The listing builds one solid part. Answer for the finished solid, in the listing's coordinates (mm). Face numbers are marked on the shaded views. A direction names the side the tool comes from. Coordinates: 2 decimals unless noted, no trailing zeros. Order: outer loops, then holes, each group sorted by start corner. A loop starts at its lowest first (then second) coordinate and runs counter-clockwise, first axis right, second up. Notation, with made-up numbers: (27, 21) -> (55, 21) arc R7 cw to (55, 30) -> close; hole circle Ø1 at (55, 55). An arc over 180 degrees is marked (long way). Return JSON: item names as keys, results as strings.
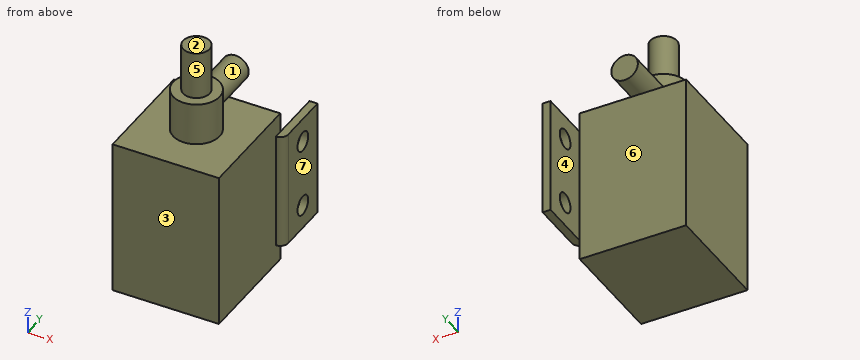
Autodesk Fusion 360 part; units mm, degrees
sketch "Sketch1" plane through (0, 0, 0) normal (0, 0, 1) x (1, 0, 0)
  line L0 (0, 0) -> (20, 0)
  line L1 (20, 0) -> (20, 21)
  line L2 (20, 21) -> (0, 21)
  line L3 (0, 21) -> (0, 0)
  dimension "d1" = 20
  dimension "d2" = 21
extrude "Extrude1" add sketch "Sketch1" along normal blind 29.5 makes body 1
sketch "Sketch2" plane through (20, 0, 0) normal (1, 0, 0) x (0, 0, -1)
  line L0 (0, 0) -> (0, 21)
  line L1 (0, 21) -> (-29.5, 21)
  line L2 (-29.5, 21) -> (-29.5, 0)
  line L3 (-29.5, 0) -> (0, 0)
  line L4 (-25.75, 21) -> (-3.75, 21)
  line L5 (-3.75, 21) -> (-3.75, 31)
  line L6 (-3.75, 31) -> (-25.75, 31)
  line L7 (-25.75, 31) -> (-25.75, 21)
  line L8 (0, 0) -> (0, 21)
  line L9 (0, 0) -> (-29.5, 0)
  circle A0 centre (-21.2, 26) radius 1.825
  circle A1 centre (-8.3, 26) radius 1.825
  line L10 (-8.3, 26) -> (-21.2, 26) construction
  point P0 (-14.75, 0)
  point P1 (-14.75, 31)
  point P2 (-14.75, 26)
  point P3 (-3.75, 26)
  dimension "d5" = 22
  dimension "d6" = 10
  dimension "d7" = 3.65
  dimension "d8" = 3.65
  dimension "d9" = 12.9
extrude "Extrude2" add sketch "Sketch2" along normal blind 1.5 separate body contours L1 L4 L5 L6 L7 makes body 2
extrude "Extrude3" add 1 faces at (20.5, 21, 11.0833) along direction (0, -1, 0) blind 1.5 on bodies 2 bodies 2 1
fillet "Fillet1" radius 1.5 1 edges at (21.5, 19.5, 14.75) on bodies 2
sketch "Sketch3" plane through (0, 0, 29.5) normal (0, 0, 1) x (1, 0, 0)
  line L0 (0, 21) -> (0, 0)
  line L1 (0, 0) -> (20, 0)
  line L2 (20, 0) -> (20, 21)
  line L3 (20, 21) -> (0, 21)
  circle A0 centre (10, 10.5) radius 4.375
  point P0 (20, 10.5)
  point P1 (10, 0)
  dimension "d15" = 8.75
extrude "Extrude4" add sketch "Sketch3" along normal blind 8 contours A0 bodies 2
sketch "Sketch4" plane through (0, 0, 37.5) normal (0, 0, 1) x (1, 0, 0)
  circle A0 centre (10, 10.5) radius 4.375
  circle A1 centre (10, 10.5) radius 2.5
  dimension "d18" = 5
extrude "Extrude5" add sketch "Sketch4" along normal blind 9 contours A1 bodies 2
ref_plane "WorkPlane1" through (10, 10.5, 14.75) normal (0, 1, 0) x (-1, 0, 0)
sketch "Sketch5" plane through (10, 10.5, 14.75) normal (0, 1, 0) x (1, 0, 0)
  line L0 (-4.375, -22.75) -> (4.375, -22.75)
  circle A0 centre (0, -18.75) radius 2.5
  point P0 (0, -22.75)
  dimension "d21" = 5
  dimension "d22" = 4
extrude "Extrude6" add sketch "Sketch5" along normal blind 13.375 bodies 2
equation "d8 = d7"
equation "d23 = ( 8.75 / 2 ) * 1 mm + 9 mm"
Item 1: Find the intervals of material crossed by probe 1 along X at (y, z) = (14, 23); probe 2 along Z at (x, y) = (13, 10.5); probe 3 along Z at (x, y) = (5, 16), in increasing order.
Answer list:
{"probe 1": "0 to 20", "probe 2": "0 to 37.5", "probe 3": "0 to 29.5"}
Item 2: Flat-ended cylindrical pins translate along their axes: pin 1 (1.2 mm diameter, centred on x = 20.5, y = 23.5, fed in from +Z); pin 2 (6 mm diameter, centred on x = 14.5, z = 37, fed in from -Y); pin 3 (8 mm diameter, centred on y = 26.5, z = 19, fed in from -X). Find the tip coordinate at first contact, or state that the pin passes through.
Answer list:
{"pin 1": "z = 25.75", "pin 2": "y = 6.39", "pin 3": "x = 20"}
Item 3: The part is cut by section C-C on x = 10. Determine the outline of the cut face in (y, z) (3 decimals), plus the area to 4 significant figures.
Answer list:
{"outline": "(0, 0) -> (21, 0) -> (21, 29.5) -> (14.875, 29.5) -> (14.875, 31) -> (23.875, 31) -> (23.875, 36) -> (14.875, 36) -> (14.875, 37.5) -> (13, 37.5) -> (13, 46.5) -> (8, 46.5) -> (8, 37.5) -> (6.125, 37.5) -> (6.125, 29.5) -> (0, 29.5) -> close", "area": "779.5 mm2"}
Item 4: The part is cut by section D-D on y = 10.5. Determine the outline of the cut face in (x, z) (3 decimals), plus the area to 3 significant figures.
Answer list:
{"outline": "(0, 0) -> (20, 0) -> (20, 29.5) -> (14.375, 29.5) -> (14.375, 37.5) -> (12.5, 37.5) -> (12.5, 46.5) -> (7.5, 46.5) -> (7.5, 37.5) -> (5.625, 37.5) -> (5.625, 29.5) -> (0, 29.5) -> close", "area": "705 mm2"}
Item 5: Which of the six approach directions +Z, -Z, +X, -X, +Y, -Y give full straight-line access (tool end or side, diameter ignored) to the marked faces 4, 5, 6 and 7?
Answer list:
{"face 4": "+Z, -Z, -X, +Y", "face 5": "+Z", "face 6": "-Z, -X, +Y", "face 7": "+Z, -Z, +X, +Y, -Y"}
Item 6: The part is cut by section A-A on y = 26. Determine the outline of the cut face in (x, z) (3 decimals), plus the area to 4 significant figures.
Answer list:
{"outline": "(20, 3.75) -> (21.5, 3.75) -> (21.5, 6.475) -> (20, 6.475) -> close; (20, 10.125) -> (21.5, 10.125) -> (21.5, 19.375) -> (20, 19.375) -> close; (20, 23.025) -> (21.5, 23.025) -> (21.5, 25.75) -> (20, 25.75) -> close", "area": "22.05 mm2"}
Item 7: Determine the mould class of the marked faces 1, 2 and 3 for opening direction Z: pulls with the +Z half, pulls with the -Z half, needs draft (parallel to the pull), parting line crosses it, or undercut.
Answer list:
{"face 1": "undercut", "face 2": "pulls with the +Z half", "face 3": "needs draft"}
